CAD build for the part. Positions are in the model's coordinates, mm. Round coordinates to 2 decimals unless told otherwise and drop trailing zeros. Loops run counter-clockwise (first coordinate to the right, second up) from the corner with the lowest first, then second, coordinate; pieces in that order, holes last. Notation, with made-up numbers: M 30,10 L 50,10 A26 cw 50,36 Z; hole C 41.25,14 d5. An arc over 180 degrees is marked long. Put each result on its own line as item: value. Start each with the question number.
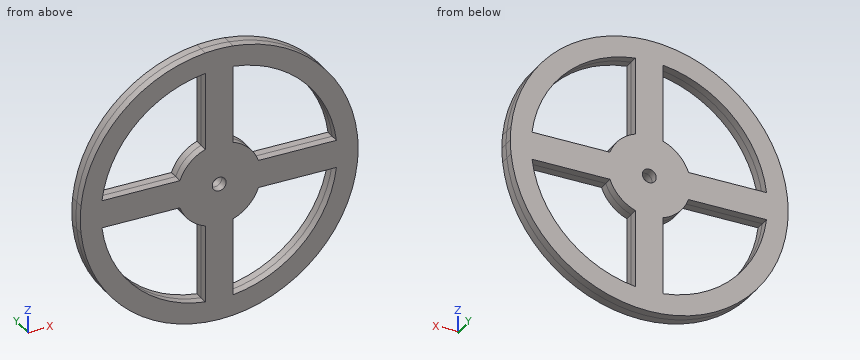
from build123d import *

# Parameters (mm, degrees)
F0_R     = 12.7
F1_DEPTH = 14.986


# Not quite as in the source:
# - a feature names something its author has since deleted; it is built from what else it names


with BuildPart() as f1:
    # F0 (on Front) → F1 (new body, symmetric)
    with BuildSketch(Plane.XZ):
        with BuildLine():
            ThreePointArc((252.7268090251, -25.4), (253.68150257, -12.7159448652), (254, 0))
            ThreePointArc((254, 0), (253.68150257, 12.7159448652), (252.7268090251, 25.4))
            ThreePointArc((252.7268090251, 25.4), (179.6051224214, 179.6051224214), (25.4, 252.7268090251))
            ThreePointArc((25.4, 252.7268090251), (0, 254), (-25.4, 252.7268090251))
            ThreePointArc((-25.4, 252.7268090251), (-179.6051224214, 179.6051224214), (-252.7268090251, 25.4))
            ThreePointArc((-252.7268090251, 25.4), (-254, 0), (-252.7268090251, -25.4))
            ThreePointArc((-252.7268090251, -25.4), (-179.6051224214, -179.6051224214), (-25.4, -252.7268090251))
            ThreePointArc((-25.4, -252.7268090251), (-1.543e-07, -254), (25.399999693, -252.7268090559))
            ThreePointArc((25.399999693, -252.7268090559), (179.6051223123, -179.6051225305), (252.7268090251, -25.4))
        make_face()
        with BuildLine():
            ThreePointArc((-25.4, -214.4006763049), (-152.6643540582, -152.6643540582), (-214.4006763049, -25.4))
            Line((-214.4006763049, -25.4), (-71.8420489686, -25.4))
            ThreePointArc((-71.8420489686, -25.4), (-53.8815367264, -53.8815367264), (-25.4, -71.8420489686))
            Line((-25.4, -71.8420489686), (-25.4, -214.4006763049))
        make_face(mode=Mode.SUBTRACT)
        with BuildLine():
            ThreePointArc((25.399999693, -71.8420490771), (53.8815366113, -53.8815368415), (71.8420489686, -25.4))
            Line((71.8420489686, -25.4), (214.4006763049, -25.4))
            ThreePointArc((214.4006763049, -25.4), (152.6643539489, -152.6643541675), (25.399999693, -214.4006763413))
            Line((25.399999693, -214.4006763413), (25.399999693, -71.8420490771))
        make_face(mode=Mode.SUBTRACT)
        with BuildLine():
            Line((-25.4, 214.4006763049), (-25.4, 71.8420489686))
            ThreePointArc((-25.4, 71.8420489686), (-53.8815367264, 53.8815367264), (-71.8420489686, 25.4))
            Line((-71.8420489686, 25.4), (-214.4006763049, 25.4))
            ThreePointArc((-214.4006763049, 25.4), (-152.6643540582, 152.6643540582), (-25.4, 214.4006763049))
        make_face(mode=Mode.SUBTRACT)
        Circle(F0_R, mode=Mode.SUBTRACT)
        with BuildLine():
            ThreePointArc((71.8420489686, 25.4), (53.8815367264, 53.8815367264), (25.4, 71.8420489686))
            Line((25.4, 71.8420489686), (25.4, 214.4006763049))
            ThreePointArc((25.4, 214.4006763049), (152.6643540582, 152.6643540582), (214.4006763049, 25.4))
            Line((214.4006763049, 25.4), (71.8420489686, 25.4))
        make_face(mode=Mode.SUBTRACT)
    extrude(amount=F1_DEPTH, both=True)


solid = f1.part
(1) Drill centre lines: line 1 along Z through (x, y) = (0, -10); line 2 along X through (y, z) = (7, 98); line 3 along Z through (x, y) = (-99.5, -13.25). Where is each one in solid material? Low to high.
(2) Cut at B-B on y = -6.25. List the corners of the cut face in (x, z), and give its area (3 significant figures).
(3) Flat gauge pins, fed straight in: pin 1 Ø3 at (y, z) = (0.5, -194.5) entering from +X; pin 2 Ø7.5 at (y, z) = (-11, 142) entering from -X; pin 3 Ø4.5 at (y, z) = (9.5, 114) entering from +X. Where does each tip first touch, or does it go through?
(4) Cut at A-A on x = 0. List the corners of the cut face in (y, z), and give its area (3 significant figures).
(5) Cut at C-C on x = 51. List the corners of the cut face in (y, z).
(6) Cut at D-D on x = 108. List the corners of the cut face in (y, z), and give its area (3 significant figures).
Taken from the geometry:
1. line 1: -254 to -12.7, 12.7 to 254
1. line 2: -234.33 to -192.38, -25.4 to 25.4, 192.38 to 234.33
1. line 3: -233.7 to -191.61, -25.4 to 25.4, 191.61 to 233.7
2. outline: C 0,0 d508; hole M -214.4,-25.4 A215.9 ccw -25.4,-214.4 L -25.4,-71.84 A76.2 cw -71.84,-25.4 Z; hole M -214.4,25.4 L -71.84,25.4 A76.2 cw -25.4,71.84 L -25.4,214.4 A215.9 ccw Z; hole C 0,0 d25.4; hole M 25.4,-214.4 A215.9 ccw 214.4,-25.4 L 71.84,-25.4 A76.2 cw 25.4,-71.84 Z; hole M 25.4,71.84 A76.2 cw 71.84,25.4 L 214.4,25.4 A215.9 ccw 25.4,214.4 Z
2. area: 103,000 mm2
3. pin 1: x = 165.13
3. pin 2: x = -213.08
3. pin 3: x = 228.1
4. outline: M -14.99,-254 L 14.99,-254 L 14.99,-12.7 L -14.99,-12.7 Z; M -14.99,12.7 L 14.99,12.7 L 14.99,254 L -14.99,254 Z
4. area: 14,500 mm2
5. outline: M -14.99,-248.83 L 14.99,-248.83 L 14.99,-209.79 L -14.99,-209.79 Z; M -14.99,-56.62 L 14.99,-56.62 L 14.99,56.62 L -14.99,56.62 Z; M -14.99,209.79 L 14.99,209.79 L 14.99,248.83 L -14.99,248.83 Z
6. outline: M -14.99,-229.9 L 14.99,-229.9 L 14.99,-186.95 L -14.99,-186.95 Z; M -14.99,-25.4 L 14.99,-25.4 L 14.99,25.4 L -14.99,25.4 Z; M -14.99,186.95 L 14.99,186.95 L 14.99,229.9 L -14.99,229.9 Z
6. area: 4,100 mm2
